Design review of the part shown in the three views and the two pictorial views. Dimensions are in mm from the part's minimum x, y and z. A direction names the side the tool comes from. Give positions to 0.01 mm unless a question says otherwise; leave off trailing zeros. Loops run counter-clockwise (first coordinate to the right, second up) from the corner with the lowest first, then second, coordinate; pieces in that order, holes last. Notation, with made-up numbers: (-37.75, -6.5) -> (6.25, -6.5) arc R25 ccw to (6.25, 32.5) -> close; hole circle Ø8 at (76.5, 20.25). An arc over 180 degrees is marked (long way). Answer as CSV lines item,"result". Start each with the question number.
Item 1: Clearance check with flat-ended pins moving along their axes: P1, Ø8.5, axis at x = 20, y = 4, coming from the -Z side; P2, Ø20, axis at y = 27.36, z = 17.5, coming from the -X side; P3, Ø6, axis at y = 27.36, z = 17.5, coming from the -X side; P4, Ø21, axis at x = 20, y = 93.74, coming from the -Z side. State where each tip first meets the part, or that it passes through.
Item 2: Add section C-C on y = 57. State the section outline as (x, z) points.
Item 3: Add section A-A on z = 17.5. State the section outline as (x, y) points, plus the area to 3 significant figures.
Item 4: The part is to be moulded in two halves that separate along X. For the marked faces 1, 2 and 3, say which applies: +X half, -X half, draft (parallel to the pull), parting line (faces both ways), or undercut.
Item 5: Add section B-B on x = 20. State how many separate pieces and enclosed holes the cut face has, plus the area to 3 significant figures.
Item 6: Machinability: for the marked faces 4, 5 and 6, which of the approach directions +Z, -Z, +X, -X, +Y, -Y give a long, thin tool a straight path to every point of the face, cutting with its end or side? Answer none if there is none.
Item 7: Add section D-D on x = 34. State the section outline as (y, z) points.
Item 8: For L1, parallel to Y at x = 20, z = 9; L2, parallel to Y at x = 20, z = 29; L3, parallel to Y at x = 14.5, z = 5.5, list the stretches that pass through material, from the lowest coordinate up. Write a range as from..to.
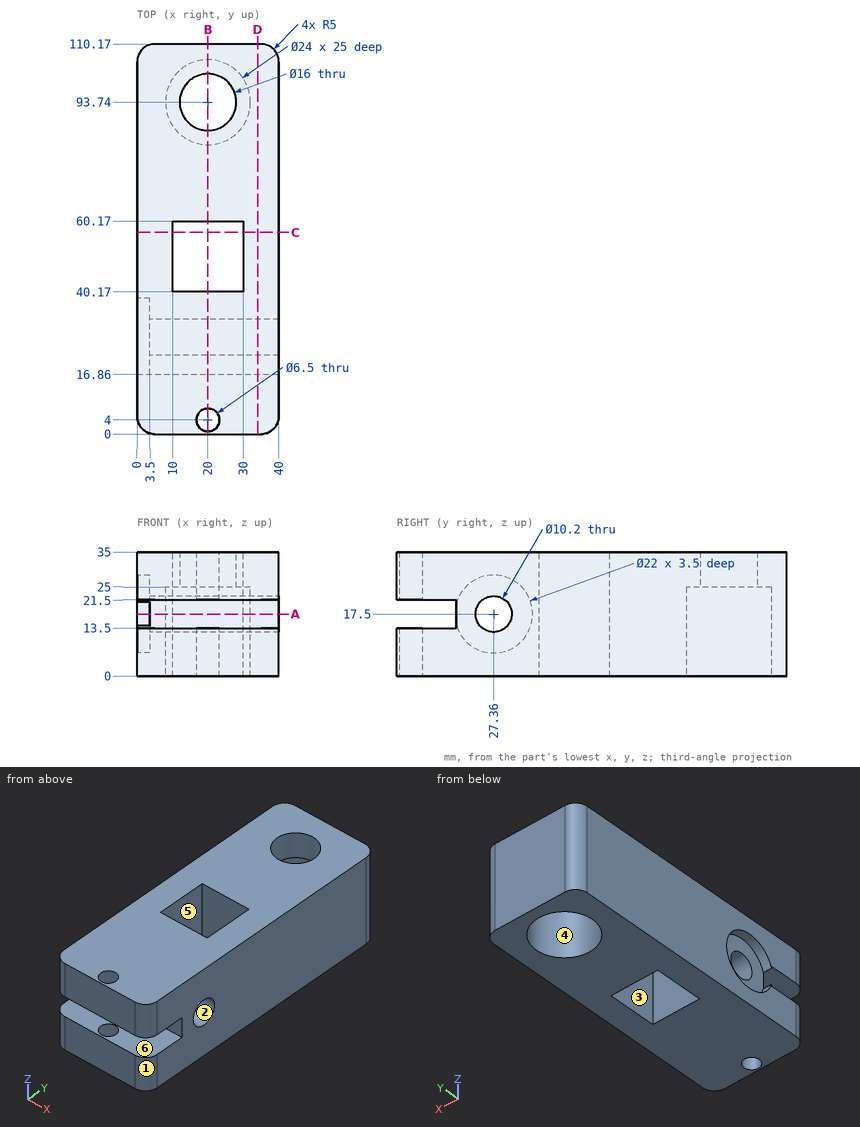
Computed values:
1,P1,"z = 0"
1,P2,"x = 3.5"
1,P3,"through"
1,P4,"z = 25"
2,outline,"(0, 0) -> (10, 0) -> (10, 35) -> (0, 35) -> close; (30, 0) -> (40, 0) -> (40, 35) -> (30, 35) -> close"
3,outline,"(0, 38.36) -> (3.5, 38.36) -> (3.5, 32.46) -> (40, 32.46) -> (40, 105.17) arc R5 ccw to (35, 110.17) -> (5, 110.17) arc R5 ccw to (0, 105.17) -> close; (3.5, 16.86) -> (40, 16.86) -> (40, 22.26) -> (3.5, 22.26) -> close; hole circle Ø24 at (20, 93.74); hole (10, 40.17) -> (30, 40.17) -> (30, 60.17) -> (10, 60.17) -> close"
3,area,"2,420 mm²"
4,face 1,"+X half"
4,face 2,"draft"
4,face 3,"undercut"
5,separate pieces,"5"
5,enclosed holes,"1"
5,area,"2,000 mm²"
6,face 4,"-Z"
6,face 5,"+Z, -Z"
6,face 6,"+X, -X, -Y"
7,outline,"(0, 0) -> (110.17, 0) -> (110.17, 35) -> (0, 35) -> (0, 21.5) -> (16.86, 21.5) -> (16.86, 13.5) -> (0, 13.5) -> close; hole circle Ø10.2 at (27.36, 17.5)"
8,L1,"0..0.75, 7.25..40.17, 60.17..81.74, 105.74..110.17"
8,L2,"0..0.75, 7.25..40.17, 60.17..85.74, 101.74..110.17"
8,L3,"0..40.17, 60.17..83.07, 104.41..110.17"
